Autodesk Inventor part; units mm, degrees
ref_plane "YZ Plane" through (0, 0, 0) normal (1, 0, 0) x (0, 1, 0)
ref_plane "XZ Plane" through (0, 0, 0) normal (0, 1, 0) x (-1, 0, 0)
ref_plane "XY Plane" through (0, 0, 0) normal (0, 0, 1) x (1, 0, 0)
sketch "Sketch1" plane through (0, 0, 0) normal (1, 0, 0) x (0, 1, 0)
  line L0 (-30, 7.5) -> (30, 7.5)
  line L1 (30, 7.5) -> (30, -7.5)
  line L2 (30, -7.5) -> (-30, -7.5)
  line L3 (-30, -7.5) -> (-30, 7.5)
  line L4 (-30, 7.5) -> (30, -7.5) construction
  line L5 (30, 7.5) -> (-30, -7.5) construction
  line L6 (-29, 6.5) -> (29, 6.5)
  line L7 (29, 6.5) -> (29, -6.5)
  line L8 (29, -6.5) -> (-29, -6.5)
  line L9 (-29, -6.5) -> (-29, 6.5)
  line L10 (-29, 6.5) -> (29, -6.5) construction
  line L11 (29, 6.5) -> (-29, -6.5) construction
  point P0 (0, 0)
  dimension "d0" = 60
  dimension "d1" = 15
  dimension "d2" = 58
  dimension "d3" = 13
extrude "Extrusion1" add sketch "Sketch1" along normal blind 800
sketch "Sketch2" plane through (0, 30, 7.5) normal (0, 1, 0) x (1, 0, 0)
  circle A0 centre (20, 7.5) radius 2.75
  circle A1 centre (780, 7.5) radius 2.75
  circle A2 centre (760, 7.5) radius 2.75
  circle A3 centre (40, 7.5) radius 2.75
  line L0 (0, 0) -> (0, 15)
  line L1 (0, 0) -> (800, 0)
  line L2 (800, 15) -> (800, 0)
  point P0 (0, 7.5)
  dimension "d6" = 5.5
  dimension "d7" = 5.5
  dimension "d8" = 5.5
  dimension "d9" = 5.5
  dimension "d10" = 20
  dimension "d11" = 20
  dimension "d12" = 7.5
  dimension "d13" = 7.5
  dimension "d14" = 7.5
  dimension "d15" = 7.5
  dimension "d16" = 20
  dimension "d17" = 20
extrude "Extrusion2" cut sketch "Sketch2" against normal blind 800
sketch "Sketch3" plane through (0, -30, 7.5) normal (0, 0, 1) x (1, 0, 0)
  circle A0 centre (50, 30) radius 20
  line L0 (0, 0) -> (0, 60)
  line L1 (0, 0) -> (800, 0)
  circle A1 centre (130, 30) radius 20
  circle A2 centre (210, 30) radius 20
  circle A3 centre (290, 30) radius 20
  circle A4 centre (370, 30) radius 20
  circle A5 centre (450, 30) radius 20
  circle A6 centre (530, 30) radius 20
  circle A7 centre (610, 30) radius 20
  circle A8 centre (690, 30) radius 20
  circle A9 centre (770, 30) radius 20
  point P0 (0, 30)
  dimension "d20" = 40
  dimension "d21" = 50
  dimension "d22" = 30
  dimension "d25" = 80
extrude "Extrusion3" cut sketch "Sketch3" against normal blind 100
properties part number "Bumper Plate" material "Aluminum 6061"
Check sheet for the modelled part. Datum: model origin and axes. Units: mm. A direction names the side the tool comes from. Round coordinates to 2 decimals unless told otherwise and drop trailing zeros. Write each loop counter-clockwise with the first axis right and the second up, starting at its lowest first coordinate (ties: lowest second). Pieces come first, ordered by that corner, then holes. Notation, with made-up numbers: M -21,53 L 5,53 A38 ccw 5,92 Z; hole C -30,54 d3. An arc over 180 degrees is marked long. Write item = value, one per line. Start each with the question number.
1. Scan lines: line 1 (Y direction, x = 628, z = -5.75); line 2 (Z direction, x = 32, y = 26); line 3 (Y direction, x = 130, z = 7.25). Record each from-to range of solid material in increasing order. Write a range as [from, to].
2. Release check for a two-part mould opening along Y. For faces 3 (the cylindrical face through (468.475, -7.66, 7.007)), 4 (the flat face through (394, 30, 0)), 5 (the flat face through (800, -5, -7)) record: pulls with the +Y half, pulls with the -Y half, needs draft (parallel to the pull), parting line crosses it, or undercut.
3. Section check A-A, the plane x = 450. Record the cut outline in (y, z), then the cut area to 3 significant figures.
4. Tool access check on faces 1 (the cylindrical face through (388.475, -7.66, -6.993)), 2 (the flat face through (483, 0, -6.5)). Record the directions out of +Z, -Z, +X, -X, +Y, -Y that give a thin tool (end or side, any length) a straight path to the whole face; none if there is none.
5. Gauge pin test, flat ends, axial feed: pin 1 (5 mm diameter, centred on x = 40, z = 0, fed in from +Y); pin 2 (6.5 mm diameter, centred on x = 20, z = 0, fed in from -Y). Record the tip position at first contact, or that the pin passes through.
Results found:
q1.line_1 = [-30, -29], [29, 30]
q1.line_2 = [-7.5, -6.5], [6.5, 7.5]
q1.line_3 = [-30, -20], [20, 30]
q2.face_3 = undercut
q2.face_4 = pulls with the +Y half
q2.face_5 = needs draft
q3.outline = M -30,-7.5 L -20,-7.5 L -20,-6.5 L -29,-6.5 L -29,6.5 L -20,6.5 L -20,7.5 L -30,7.5 Z; M 20,-7.5 L 30,-7.5 L 30,7.5 L 20,7.5 L 20,6.5 L 29,6.5 L 29,-6.5 L 20,-6.5 Z
q3.area = 66.0 mm^2
q4.face_1 = +Z, -Z
q4.face_2 = +X, -X
q5.pin_1 = through
q5.pin_2 = -30
